Source: CAD feature listing. Evaluate the final solid. Frame: model axes, mm. A direction names the side the tool comes from. Round coordinates to 2 decimals unless told otherwise and drop trailing zeros. Order: outer loops, then holes, each group sorted by start corner. A loop starts at its lowest first (then second) coordinate and runs counter-clockwise, first axis right, second up. Notation, with made-up numbers: M -37,-1.75 L -31,-1.75 A15 ccw -31,20.25 Z; hole C -4,-30.75 d2. An arc over 180 degrees is marked long. Answer in a Markdown table with one row per item. Add a question column.
```python
from build123d import *

# Parameters (mm, degrees)
F0_W     = 100
F0_H     = 30
F1_DEPTH = 3.5
F3_DEPTH = 3.501
F4_W     = 6
F4_H     = 4
F5_DEPTH = 3.501


with BuildPart() as f1:
    # F0 (on Front) → F1 (new body)
    with BuildSketch(Plane.XZ):
        Rectangle(F0_W, F0_H)
    extrude(amount=F1_DEPTH)

    # F2 (on face) → F3 (cut, through all)
    with BuildSketch(Plane.XZ.offset(3.5)):
        with BuildLine():
            ThreePointArc((-44.8, -11.4), (-46.4, -9.8), (-48, -11.4))
            Line((-48, -11.4), (-44.8, -11.4))
        make_face()
        with BuildLine():
            Line((-44.8, -11.4), (-48, -11.4))
            ThreePointArc((-48, -11.4), (-46.4, -13), (-44.8, -11.4))
        make_face()
        with BuildLine():
            Line((-23.6, -11.4), (-23.6, -13))
            ThreePointArc((-23.6, -13), (-22.4686291501, -12.5313708499), (-22, -11.4))
            Line((-22, -11.4), (-23.6, -11.4))
        make_face()
        with BuildLine():
            ThreePointArc((-25.2, -11.4), (-24.7313708499, -12.5313708499), (-23.6, -13))
            Line((-23.6, -13), (-23.6, -11.4))
            Line((-23.6, -11.4), (-25.2, -11.4))
        make_face()
        with BuildLine():
            Line((-25.2, -11.4), (-23.6, -11.4))
            Line((-23.6, -11.4), (-22, -11.4))
            ThreePointArc((-22, -11.4), (-23.6, -9.8), (-25.2, -11.4))
        make_face()
        with BuildLine():
            ThreePointArc((1.6, -11.4), (0, -9.8), (-1.6, -11.4))
            ThreePointArc((-1.6, -11.4), (0, -13), (1.6, -11.4))
        make_face()
    extrude(amount=-F3_DEPTH, mode=Mode.SUBTRACT)

    # F4 (on face) → F5 (cut, through all)
    with BuildSketch(Plane.XZ.offset(3.5)):
        Polygon((-34, 15), (-40, 15), (-40, 8), (-34, 8), (-34, 12), align=None)
        with Locations((-31, 10)):
            Rectangle(F4_W, F4_H)
        Polygon((1, 15), (-5, 15), (-5, 8), (1, 8), (1, 12), align=None)
        with Locations((4, 10)):
            Rectangle(F4_W, F4_H)
        Polygon((36, 15), (30, 15), (30, 8), (36, 8), (36, 12), align=None)
        with Locations((39, 10)):
            Rectangle(F4_W, F4_H)
    extrude(amount=-F5_DEPTH, mode=Mode.SUBTRACT)


solid = f1.part
```
(1) Cut plane C-C (x = -36). Return loops of the section in (y, z).
(2) Draft query along X for faces 4 (the face through (-1, -2, -15)), 5 (the face through (42, -2, 10)), 6 (the face through (-50, -2, 0)). Return one class per face: +X half, -X half, draft (parallel to the pull), parting line (faces both ways), or undercut.
(3) Line query: line 1 (X direction, y = -1, z = -11.25); line 2 (X direction, y = -3.1, z = 12.5); line 3 (Z direction, x = -46.4, y = -1.05). Output: solid intervals per line, ascending. Write a range as from..to.
(4) Cut plane B-B (y = -0.7). Return loops of the section in (x, z).
(5) Access query for faces 1 (the face through (-28, -2, 10)), 2 (the face through (15, -2, 15)), 3 (the face through (1, -2, 13)). Directions: +Z, -Z, +X, -X, +Y, -Y. A direction counts if a zero-diameter tool reaches every point of the face in a straight line with its end or side. Return the directions, or none.
(6) Pin query (flat end, axial travel): pin 1 (3 mm diameter, centred on x = 0, z = -11.4, fed in from +Y); pin 2 (1 mm diameter, centred on x = -36, y = -2, fed in from +Z). Return the tip coordinate at first contact, or that it passes through.
(7) Cut plane A-A (x = -46.4). Return loops of the section in (y, z).
Answer list:
| question | item | result |
|---|---|---|
| 1 | outline | M -3.5,-15 L 0,-15 L 0,8 L -3.5,8 Z |
| 2 | face 4 | draft |
| 2 | face 5 | undercut |
| 2 | face 6 | -X half |
| 3 | line 1 | -50..-47.99, -44.81..-25.19, -22.01..-1.59, 1.59..50 |
| 3 | line 2 | -50..-40, -34..-5, 1..30, 36..50 |
| 3 | line 3 | -15..-13, -9.8..15 |
| 4 | outline | M -50,-15 L 50,-15 L 50,15 L 36,15 L 36,12 L 42,12 L 42,8 L 30,8 L 30,15 L 1,15 L 1,12 L 7,12 L 7,8 L -5,8 L -5,15 L -34,15 L -34,12 L -28,12 L -28,8 L -40,8 L -40,15 L -50,15 Z; hole C -46.4,-11.4 d3.2; hole C -23.6,-11.4 d3.2; hole C 0,-11.4 d3.2 |
| 5 | face 1 | +Y, -Y |
| 5 | face 2 | +Z, +X, -X, +Y, -Y |
| 5 | face 3 | +Z, +Y, -Y |
| 6 | pin 1 | through |
| 6 | pin 2 | z = 8 |
| 7 | outline | M -3.5,-15 L 0,-15 L 0,-13 L -3.5,-13 Z; M -3.5,-9.8 L 0,-9.8 L 0,15 L -3.5,15 Z |
